```python
from build123d import *

# Parameters (mm, degrees)
F0_R     = 7.5
F1_DEPTH = 22
F2_R     = 8
F3_DEPTH = 20
F5_DEPTH = 22.001
F6_R     = 3.25
F7_DEPTH = 4


with BuildPart() as f1:
    # F0 (on Front) → F1 (new body)
    with BuildSketch(Plane.XZ):
        Circle(F0_R)
    extrude(amount=-F1_DEPTH)

    # F2 (on face) → F3 (cut)
    with BuildSketch(Plane(origin=(0, 22, 0), x_dir=(-1, 0, 0), z_dir=(0, 1, 0))):
        Circle(F2_R)
        Polygon((3.695042, 6.4), (7.390083, 0), (3.695042, -6.4), (-3.695042, -6.4), (-7.390083, 0), (-3.695042, 6.4), align=None, mode=Mode.SUBTRACT)
    extrude(amount=-F3_DEPTH, mode=Mode.SUBTRACT)

    # F4 (on face) → F5 (cut, through all)
    with BuildSketch(Plane.XZ):
        with BuildLine():
            Line((2.244994, 2.35), (-2.244994, 2.35))
            ThreePointArc((-2.244994, 2.35), (0, -3.25), (2.244994, 2.35))
        make_face()
    extrude(amount=-F5_DEPTH, mode=Mode.SUBTRACT)

    # F6 (on face) → F7 (cut)
    with BuildSketch(Plane.XZ):
        Circle(F6_R)
    extrude(amount=-F7_DEPTH, mode=Mode.SUBTRACT)


solid = f1.part
```
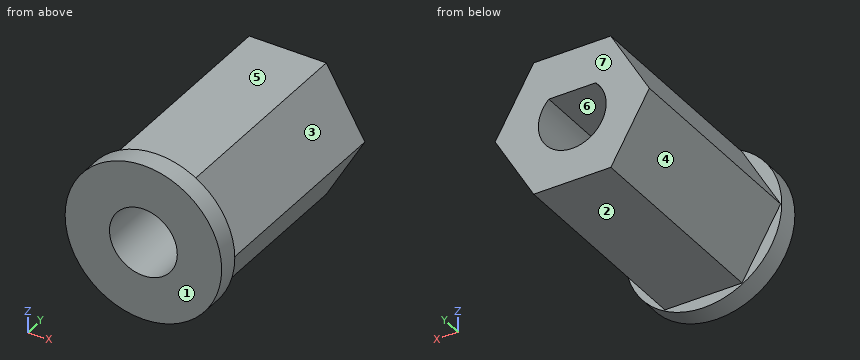
Read the model definition and answer for the solid it produces. Units are mm, in the model's axes. Face numbers are marked on the shaded views. A direction names the side the tool comes from. Give positions to 0.01 mm unless a question says otherwise; leave off trailing zeros. Order: outer loops, then holes, each group sorted by start corner. A loop starts at its lowest first (then second) coordinate and runs counter-clockwise, first axis right, second up. Notation, with made-up numbers: (47.25, 80.5) -> (77.25, 80.5) arc R23 cw to (77.25, 107.5) -> close; hole circle Ø9 at (80, -35.5). An arc over 180 degrees is marked (long way). One line per item, written item: value. Start each with the question number.
(1) Straight lines are drawn through the part: L1, parallel to Z at x = 0, y = 16.25; L2, parallel to Z at x = -3, y = 13.75; L3, parallel to Y at x = 1.5, z = 2.5. For each, find the intervals that lie inside material, in ascending order.
(2) The part is cut by section B-B (x = 0). Determine the outline of the cut face in (y, z).
(3) A tool of negligible diameter and unlimited length cuts with its end or side. For the marked faces 1, 2 and 3, from which of +Z, -Z, +X, -X, +Y, -Y can it reach the whole face along a straight path? Write none if from no direction.
(4) For a pull along Z with two mould halves and no side action, classify the marked faces 4, 5, 6 and 7 as released by +Z, released by -Z, zero draft, split by the parting line, or undercut.
(5) Flat-ended cylindrical pins translate along their axes: P1, Ø2, axis at x = 0, y = 11, coming from the +Z side; P2, Ø3, axis at y = 18, z = -2, coming from the -X side; P3, Ø8, axis at y = 19.5, z = -2, coming from the +X side. Find the tip coordinate at first contact, or state that the pin passes through.
(6) The part is cut by section C-C (z = -0.75). Determine the outline of the cut face in (x, y), and give its area (3 significant figures).
(7) The part is cut by section A-A (y = 14.5). Determine the outline of the cut face in (x, z) (3 decimals).
(8) The part is cut by section D-D (x = 4.25). Determine the outline of the cut face in (y, z), and give its area (3 significant figures).
Taken from the geometry:
1. L1: -6.4 to -3.25, 2.35 to 6.4
1. L2: -6.4 to -1.25, 1.25 to 6.4
1. L3: 4 to 22
2. outline: (0, -7.5) -> (2, -7.5) -> (2, -6.4) -> (22, -6.4) -> (22, -3.25) -> (0, -3.25) -> close; (0, 3.25) -> (4, 3.25) -> (4, 2.35) -> (22, 2.35) -> (22, 6.4) -> (2, 6.4) -> (2, 7.5) -> (0, 7.5) -> close
3. face 1: +Z, -Z, +X, -X, -Y
3. face 2: -Z, +X, -X, +Y
3. face 3: +Z, +X, +Y
4. face 4: released by -Z
4. face 5: released by +Z
4. face 6: undercut
4. face 7: zero draft
5. P1: z = 6.4
5. P2: x = -7.1
5. P3: x = 7.39
6. outline: (-7.46, 0) -> (-3.16, 0) -> (-3.16, 22) -> (-6.96, 22) -> (-6.96, 2) -> (-7.46, 2) -> close; (3.16, 0) -> (7.46, 0) -> (7.46, 2) -> (6.96, 2) -> (6.96, 22) -> (3.16, 22) -> close
6. area: 169 mm^2
7. outline: (-7.39, 0) -> (-3.695, -6.4) -> (3.695, -6.4) -> (7.39, 0) -> (3.695, 6.4) -> (-3.695, 6.4) -> close; hole (-2.245, 2.35) arc R3.25 ccw (long way) to (2.245, 2.35) -> close
8. outline: (0, -6.18) -> (2, -6.18) -> (2, -5.44) -> (22, -5.44) -> (22, 5.44) -> (2, 5.44) -> (2, 6.18) -> (0, 6.18) -> close
8. area: 242 mm^2
